Verification items for this drawing (mm, ordinates from the low corner). Coordinates: 2 decimals unless noted, no trailing zeros. Order: outer loops, then holes, each group sorted by start corner. A loop starts at its lowest first (then second) coordinate and runs counter-clockwise, first axis right, second up.
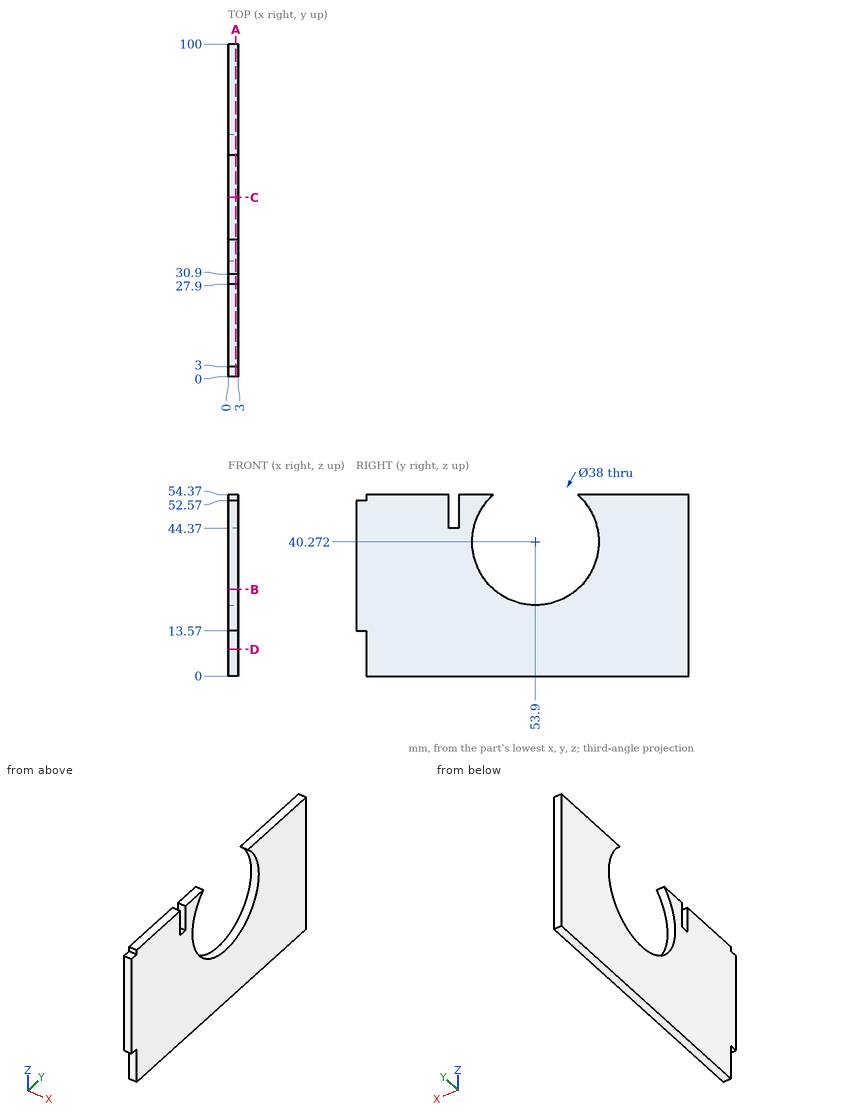
(1) Cross-section at D-D (z = 8). Enter the section's corners in (x, y).
Filled in:
outline: (0, 3) - (3, 3) - (3, 100) - (0, 100) - close
(2) Cross-section at A-A (x = 2.35). Enter the section's corners in (y, z), and give its area (3 significant figures).
Filled in:
outline: (0, 13.57) - (3, 13.57) - (3, 0) - (100, 0) - (100, 54.37) - (66.64, 54.37) arc R19 cw (long way) to (41.16, 54.37) - (30.9, 54.37) - (30.9, 44.37) - (27.9, 44.37) - (27.9, 54.37) - (3, 54.37) - (3, 52.57) - (0, 52.57) - close
area: 4,310 mm2
(3) Thickness scan on probe 1 along Y at (x, z) = (1.55, 52.5); probe 2 along Z at (x, y) = (0.5, 70); probe 3 along Y at (x, z) = (1.6, 39). Record the ranges inside material, lowest first.
Filled in:
probe 1: y = 0 to 27.9, 30.9 to 39.36, 68.44 to 100
probe 2: z = 0 to 30.18, 50.36 to 54.37
probe 3: y = 0 to 34.94, 72.86 to 100
(4) Cross-section at C-C (y = 53.9). Enter the section's corners in (x, z).
Filled in:
outline: (0, 0) - (3, 0) - (3, 21.27) - (0, 21.27) - close
(5) Go/stop test with a flat-tipped pin: P1, Ø1.5, axis at x = 1.5, y = 1.5, coming from the +Z side. Record where the tip stops, or that it passes through.
Filled in:
P1: stops at z = 52.57
(6) Cross-section at B-B (z = 26). Enter the section's corners in (x, y), and give its area (3 significant figures).
Filled in:
outline: (0, 0) - (3, 0) - (3, 41.36) - (0, 41.36) - close; (0, 66.44) - (3, 66.44) - (3, 100) - (0, 100) - close
area: 225 mm2
